Could you check a few things on this model? Use its own coordinates, in mm. Face numbers are marked on the shaded views. A direction names the side the tool comes from. Give positions to 0.01 mm unless a question says otherwise; leave off trailing zeros. Loops run counter-clockwise (first coordinate to the right, second up) from the corner with the lowest first, then second, coordinate; pieces in that order, holes last. Notation, with made-up numbers: (-9, 31.25) - (37, 31.25) arc R30 ccw to (37, 68.25) - close; hole circle Ø5 at (42, -36.75). An arc over 180 degrees is marked (long way). Answer in a Markdown table with one row per item. Add a question column.
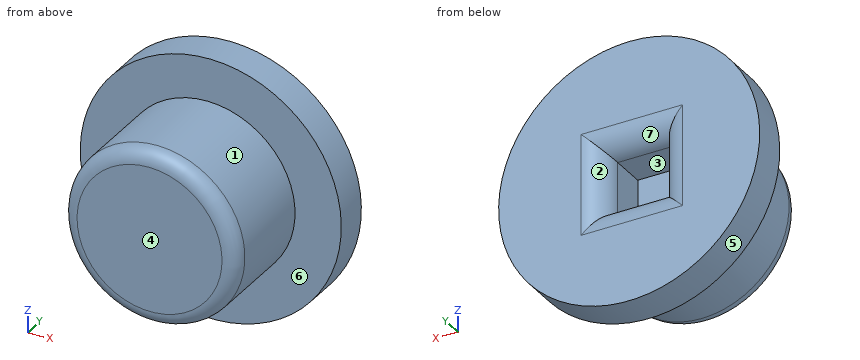
```python
from build123d import *

# Parameters (mm, degrees)
SKETCH_1_R          = 3
EXTRUDE_1_DEPTH     = 3.5
SKETCH_2_R          = 4.5
EXTRUDE_2_DEPTH     = 1.2
SKETCH_4_W          = 1.9
SKETCH_4_H          = 1.9
CUT_EXTRUDE_1_DEPTH = 2
FILLET_1_R          = 0.5
FILLET_2_R          = 0.8


with BuildPart() as part:
    # 草图1 → 凸台-拉伸1 (new body)
    with BuildSketch(Plane(origin=(0, 0, 0), x_dir=(1, 0, 0), z_dir=(0, 1, 0))):
        with Locations(Location((0, 0, 0), (0, 0, 270))):
            Circle(SKETCH_1_R)
    extrude(amount=EXTRUDE_1_DEPTH)

    # 草图2 → 凸台-拉伸2 (add)
    with BuildSketch(Plane(origin=(0, 3.5, 0), x_dir=(1, 0, 0), z_dir=(0, 1, 0))):
        with Locations(Location((0.094879954, 0.012027373, 0), (0, 0, 270))):
            Circle(SKETCH_2_R)
    extrude(amount=EXTRUDE_2_DEPTH)

    # 草图4 → 切除-拉伸1 (cut)
    with BuildSketch(Plane(origin=(0, 4.7, 0), x_dir=(1, 0, 0), z_dir=(0, 1, 0))):
        Rectangle(SKETCH_4_W, SKETCH_4_H)
    extrude(amount=-CUT_EXTRUDE_1_DEPTH, mode=Mode.SUBTRACT)

    # 圆角1
    fillet_1_edges = [part.edges().sort_by_distance(p)[0] for p in [
        (0, 0, -3),
    ]]
    fillet(fillet_1_edges, radius=FILLET_1_R)

    # 圆角2
    fillet_2_edges = [part.edges().sort_by_distance(p)[0] for p in [
        (-0.95, 4.7, 0),
        (0, 4.7, 0.95),
        (0.95, 4.7, 0),
        (0, 4.7, -0.95),
    ]]
    fillet(fillet_2_edges, radius=FILLET_2_R)


solid = part.part
```
(1) Please list where these lines run through material, in increasing order: line 1 (Y direction, x = 4.25, z = 0.25); line 2 (X direction, y = 2.75, z = -0.25); line 3 (X direction, y = 4.3, z = 0.25).
(2) I want a section at B-B on z = 0. Please give me the cut outline in (x, y), then the cut area to 3 significant figures.
(3) I want a section at A-A on y = 2.85. Please give me the cut outline in (x, z).
(4) I want a section at C-C on y = 1.4. Please give me the cut outline in (x, z).
(5) On a 3-axis mill with a long thin cutter (end or side, diameter ignored), from which of +Z, -Z, +X, -X, +Y, -Y can I reach the whole of each face in a straight line? I mean the marked faces 5, 6 and 7. Say none if no direction works.
(6) I want a section at D-D on y = 4.45. Please give me the cut outline in (x, z).
(7) For pin 1 Ø2 at (y, z) = (0.5, 1.5) entering from +X; pin 2 Ø1.3 at (y, z) = (3, 0) entering from +X; pin 3 Ø2 at (y, z) = (1.5, 1) entering from -X; pin 4 Ø2 at (y, z) = (1.5, -3.5) entering from -X, each with a flat end and sliding along its axis, tell me the tip position at first contact or that it passes through.
(8) We'd pull the mould along Z, two halves only. Please class the marked faces 1, 2, 3 and 4: pulls with the +Z half, pulls with the -Z half, needs draft (parallel to the pull), parting line crosses it, or undercut.
Reported:
| question | item | result |
|---|---|---|
| 1 | line 1 | 3.5 to 4.7 |
| 1 | line 2 | -2.99 to -0.95, 0.95 to 2.99 |
| 1 | line 3 | -4.4 to -1.06, 1.06 to 4.59 |
| 2 | outline | (-4.41, 3.5) - (-3, 3.5) - (-3, 0.5) arc R0.5 ccw to (-2.5, 0) - (2.5, 0) arc R0.5 ccw to (3, 0.5) - (3, 3.5) - (4.59, 3.5) - (4.59, 4.7) - (1.75, 4.7) arc R0.8 ccw to (0.95, 3.9) - (0.95, 2.7) - (-0.95, 2.7) - (-0.95, 3.9) arc R0.8 ccw to (-1.75, 4.7) - (-4.41, 4.7) - close |
| 2 | area | 27.6 mm² |
| 3 | outline | circle Ø6 at (0, 0); hole (-0.95, -0.95) - (0.95, -0.95) - (0.95, 0.95) - (-0.95, 0.95) - close |
| 4 | outline | circle Ø6 at (0, 0) |
| 5 | face 5 | +Y, -Y |
| 5 | face 6 | -Y |
| 5 | face 7 | +Y |
| 6 | outline | circle Ø9 at (0.09, -0.01); hole (-1.17, -1.17) - (1.17, -1.17) - (1.17, 1.17) - (-1.17, 1.17) - close |
| 7 | pin 1 | x = 2.96 |
| 7 | pin 2 | x = 4.59 |
| 7 | pin 3 | x = -3 |
| 7 | pin 4 | x = -1.66 |
| 8 | face 1 | parting line crosses it |
| 8 | face 2 | undercut |
| 8 | face 3 | undercut |
| 8 | face 4 | needs draft |
